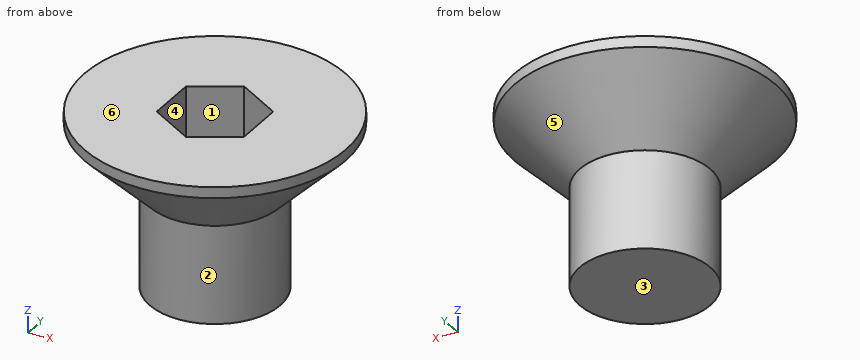
Autodesk Inventor part; units mm, degrees
ref_plane "YZ Plane" through (0, 0, 0) normal (1, 0, 0) x (0, 1, 0)
ref_plane "XZ Plane" through (0, 0, 0) normal (0, 1, 0) x (-1, 0, 0)
ref_plane "XY Plane" through (0, 0, 0) normal (0, 0, 1) x (1, 0, 0)
sketch "スケッチ1" plane through (0, 0, 0) normal (0, 0, 1) x (1, 0, 0)
  circle A0 centre (0, 0) radius 1.5
  dimension "d0" = 3
extrude "押し出し1" add sketch "スケッチ1" along normal blind 4
thread "ねじ1"
sketch "スケッチ2" plane through (0, 0, 4) normal (0, 0, 1) x (1, 0, 0)
  circle A0 centre (0, 0) radius 3
  dimension "d5" = 6
extrude "押し出し2" add sketch "スケッチ2" against normal blind 1.75
chamfer "面取り1" distance 1.5 angle 45 1 edges at (-3, 0, 2.25)
sketch "スケッチ3" plane through (0, 0, 4) normal (0, 0, 1) x (1, 0, 0)
  line L0 (0, 1.1547) -> (1, 0.5774)
  line L1 (1, 0.5774) -> (1, -0.5774)
  line L2 (1, -0.5774) -> (0, -1.1547)
  line L3 (0, -1.1547) -> (-1, -0.5774)
  line L4 (-1, -0.5774) -> (-1, 0.5774)
  line L5 (-1, 0.5774) -> (0, 1.1547)
  point P0 (0, 0)
  point P1 (0, 0)
  dimension "d11" = 2
extrude "押し出し3" cut sketch "スケッチ3" against normal blind 1.5
properties part number "m3皿ネジ4" material "鉄 灰色"
Build history of the part. All positions in model axes, mm. Face numbers are marked on the shaded views. A direction names the side the tool comes from. Round coordinates to 2 decimals unless told otherwise and drop trailing zeros. Write each loop counter-clockwise with the first axis right and the second up, starting at its lowest first coordinate (ties: lowest second). Pieces come first, ordered by that corner, then holes. Notation, with made-up numbers: M 73.25,24.5 L 123.25,24.5 A15 cw 123.25,32.5 Z; hole C -15,0 d10. An arc over 180 degrees is marked long. Answer in a Markdown table with one row per item.
1. Which spindle directions (+Z, -Z, +X, -X, +Y, -Y) get a long thin tool onto all of the face, cutting with end or side? Do the marked faces 1, 2 and 3. Say none if no direction does.
Geometry check:
| item | result |
|---|---|
| face 1 | +Z |
| face 2 | -Z |
| face 3 | -Z, +X, -X, +Y, -Y |
2. Flat gauge pins, fed straight in: P1, Ø1.5, axis at x = -1, z = 2, coming from the +Y side; P2, Ø1.6, axis at x = 0, y = 0, coming from the +Z side; P3, Ø0.6, axis at y = 0, z = 3, coming from the -X side. Where does each tip first touch, or does it go through?
Geometry check:
| item | result |
|---|---|
| P1 | y = 1.81 |
| P2 | z = 2.5 |
| P3 | x = -2.55 |
3. Mould opens along Y. For the marked faces 4, 5 and 6 say: +Y half, -Y half, draft (parallel to the pull), parting line (faces both ways), or undercut.
Geometry check:
| item | result |
|---|---|
| face 4 | undercut |
| face 5 | parting line |
| face 6 | draft |
4. Saw through at C-C (z = 1.7). List the corners of the cut face in (x, y).
Geometry check:
| item | result |
|---|---|
| outline | C 0,0 d3 |
5. Saw through at B-B (z = 2.8). List the corners of the cut face in (x, y), and give its area (3 significant figures).
Geometry check:
| item | result |
|---|---|
| outline | C 0,0 d4.1; hole M -1,-0.58 L 0,-1.15 L 1,-0.58 L 1,0.58 L 0,1.15 L -1,0.58 Z |
| area | 9.74 mm2 |
6. Probe L1, parallel to Y at x = -0.55, z = 2.9; L2, parallel to X at y = -0.55, z = 3.65; L3, parallel to X at y = -0.75, z = 3.4. List the from-to ranges inside material, lowest first. Write a range as [from, to].
Geometry check:
| item | result |
|---|---|
| L1 | [-2.08, -0.84], [0.84, 2.08] |
| L2 | [-2.85, -1], [1, 2.85] |
| L3 | [-2.54, -0.7], [0.7, 2.54] |
